The listing builds one solid part. Answer for the finished solid, in the listing's coordinates (mm). Face numbers are marked on the shaded views. Give positions to 0.01 mm unless a question says otherwise; leave off trailing zeros. Order: outer loops, then holes, each group sorted by start corner. A loop starts at its lowest first (then second) coordinate and runs counter-clockwise, first axis right, second up. Notation, with made-up numbers: (20.5, -4.75) - (79.5, -4.75) arc R25 ccw to (79.5, 15.25) - close; hole circle Ø5 at (62, -14). An arc over 180 degrees is marked (long way). Use a Markdown table: item, result. Add a question column.
1) Find section B-B, the plane x = -7.5. Determine the outline of the cut face in (y, z), plus the area to 3 significant figures.
2) Find section C-C, the plane y = 57. Determine the outline of the cut face in (x, z).
3) The mould has two halves that part along Y. Classify the marked faces 1, 2, 3 and 4: released by +Y, released by -Y, zero draft, split by the parting line, or undercut.
4) Flat-ended cylindrical pins translate along their axes: pin 1 (10.5 mm diameter, centred on x = -7.5, z = 17.5, fed in from +Y); pin 2 (4 mm diameter, centred on y = 140.38, z = 25, fed in from +X); pin 3 (10 mm diameter, centred on y = 114.5, z = 27.5, fed in from -X); pin 4 (10 mm diameter, centred on y = 145, z = 35, fed in from -X). Find the tip coordinate at first contact, or state that the pin passes through.
5) Straight lines are drawn through the part: line 1 (Z direction, x = 5, y = 152.5); line 2 (Z direction, x = -7.5, y = 4); line 3 (X direction, y = 150.5, z = 57.5). For each, find the intervals that lie inside material, in ascending order.
6) Find section A-A, the plane z = 50. Determine the outline of the cut face in (x, y), plus the area to 3 significant figures.
7) Find section D-D, the plane z = 32. Determine the outline of the cut face in (x, y), plus the area to 3 significant figures.
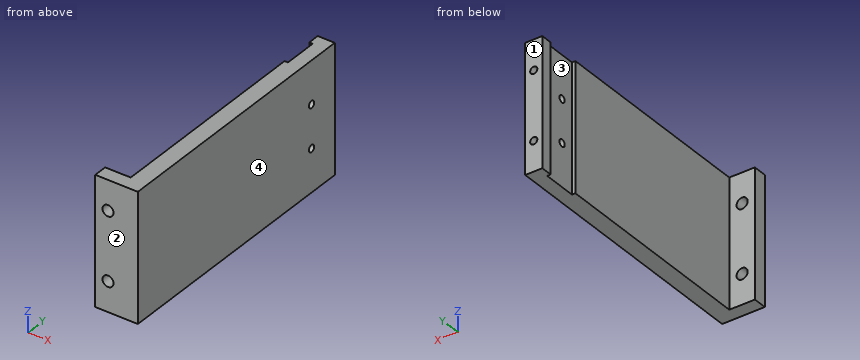
from build123d import *

# Parameters (mm, degrees)
SKETCH_1_W             = 10
SKETCH_1_H             = 159.15
EXTRUDE_1_DEPTH        = 75
HOLE_WIZARD_M5_1_D     = 4.2
HOLE_WIZARD_M5_1_DEPTH = 12.4
HOLE_WIZARD_M5_1_TIP   = 1.2618073
SKETCH_4_W             = 75
SKETCH_4_H             = 20
CUT_EXTRUDE_1_DEPTH    = 2
HOLE_WIZARD_M5_2_D     = 4.2
HOLE_WIZARD_M5_2_DEPTH = 12.4
HOLE_WIZARD_M5_2_TIP   = 1.2618073
SKETCH_7_W             = 75
SKETCH_7_H             = 8
EXTRUDE_2_DEPTH        = 15
SKETCH_8_R             = 3.25
CUT_EXTRUDE_2_DEPTH    = 9


with BuildPart() as part:
    # 草图1 → 凸台-拉伸1 (new body)
    with BuildSketch(Plane.XY):
        with Locations((5, 79.575)):
            Rectangle(SKETCH_1_W, SKETCH_1_H)
    extrude(amount=EXTRUDE_1_DEPTH)

    # M5 螺纹孔1
    with Locations(Plane(origin=(0, 159.15, 0), x_dir=(1, 0, 0), z_dir=(0, 1, 0))):
        with Locations((5, -57.5), (5, -17.5)):
            Hole(HOLE_WIZARD_M5_1_D / 2, depth=HOLE_WIZARD_M5_1_DEPTH)
            with Locations((0, 0, -(HOLE_WIZARD_M5_1_DEPTH + HOLE_WIZARD_M5_1_TIP / 2))):  # 118° drill point
                Cone(0, HOLE_WIZARD_M5_1_D / 2, HOLE_WIZARD_M5_1_TIP, mode=Mode.SUBTRACT)

    # 草图4 → 切除-拉伸1 (cut)
    with BuildSketch(Plane.ZY):
        with Locations((37.5, 142.38)):
            Rectangle(SKETCH_4_W, SKETCH_4_H)
    extrude(amount=-CUT_EXTRUDE_1_DEPTH, mode=Mode.SUBTRACT)

    # M5 螺纹孔2
    with Locations(Plane.ZY.offset(-2)):
        with Locations((25, 140.3817), (50, 140.3817)):
            Hole(HOLE_WIZARD_M5_2_D / 2, depth=HOLE_WIZARD_M5_2_DEPTH)
            with Locations((0, 0, -(HOLE_WIZARD_M5_2_DEPTH + HOLE_WIZARD_M5_2_TIP / 2))):  # 118° drill point
                Cone(0, HOLE_WIZARD_M5_2_D / 2, HOLE_WIZARD_M5_2_TIP, mode=Mode.SUBTRACT)

    # 草图7 → 凸台-拉伸2 (add)
    with BuildSketch(Plane.ZY):
        with Locations((37.5, 4)):
            Rectangle(SKETCH_7_W, SKETCH_7_H)
    extrude(amount=EXTRUDE_2_DEPTH)

    # 草图8 → 切除-拉伸2 (cut, through all)
    with BuildSketch(Plane(origin=(0, 8, 0), x_dir=(1, 0, 0), z_dir=(0, 1, 0))):
        with Locations((-7.5, -17.5)):
            Circle(SKETCH_8_R)
        with Locations((-7.5, -57.5)):
            Circle(SKETCH_8_R)
    extrude(amount=-CUT_EXTRUDE_2_DEPTH, mode=Mode.SUBTRACT)


solid = part.part
The answers:
| question | item | result |
|---|---|---|
| 1 | outline | (0, 0) - (8, 0) - (8, 14.25) - (0, 14.25) - close; (0, 20.75) - (8, 20.75) - (8, 54.25) - (0, 54.25) - close; (0, 60.75) - (8, 60.75) - (8, 75) - (0, 75) - close |
| 1 | area | 496 mm2 |
| 2 | outline | (0, 0) - (10, 0) - (10, 75) - (0, 75) - close |
| 3 | face 1 | released by +Y |
| 3 | face 2 | released by -Y |
| 3 | face 3 | undercut |
| 3 | face 4 | zero draft |
| 4 | pin 1 | y = 8 |
| 4 | pin 2 | through |
| 4 | pin 3 | x = 0 |
| 4 | pin 4 | x = 2 |
| 5 | line 1 | 0 to 15.4, 19.6 to 55.4, 59.6 to 75 |
| 5 | line 2 | 0 to 14.25, 20.75 to 54.25, 60.75 to 75 |
| 5 | line 3 | 2 to 2.9, 7.1 to 10 |
| 6 | outline | (-15, 0) - (10, 0) - (10, 138.28) - (2, 138.28) - (2, 132.38) - (0, 132.38) - (0, 8) - (-15, 8) - close; (0, 152.38) - (2, 152.38) - (2, 142.48) - (10, 142.48) - (10, 159.15) - (0, 159.15) - close |
| 6 | area | 1,640 mm2 |
| 7 | outline | (-15, 0) - (10, 0) - (10, 159.15) - (0, 159.15) - (0, 152.38) - (2, 152.38) - (2, 132.38) - (0, 132.38) - (0, 8) - (-15, 8) - close |
| 7 | area | 1,670 mm2 |
